from build123d import *

# Parameters (mm, degrees)
SKETCH1_R                            = 3.175
SKETCH1_R_2                          = 1.5875
BOSS_EXTRUDE1_DEPTH                  = 19.05
TAPPED_HOLE_FOR_4_40_HELICOIL2_D     = 3.048
TAPPED_HOLE_FOR_4_40_HELICOIL2_DEPTH = 9.6012
TAPPED_HOLE_FOR_4_40_HELICOIL2_TIP   = 0.915711583
SKETCH7_W                            = 1.190625
SKETCH7_H                            = 3.175
TAPPED_HOLE_FOR_4_40_HELICOIL3_D     = 3.048
TAPPED_HOLE_FOR_4_40_HELICOIL3_DEPTH = 9.6012
TAPPED_HOLE_FOR_4_40_HELICOIL3_TIP   = 0.915711583


with BuildPart() as part:
    # Sketch1 → Boss-Extrude1 (new body)
    with BuildSketch(Plane(origin=(0, 0, 0), x_dir=(1, 0, 0), z_dir=(0, 1, 0))):
        with Locations(Location((0, 0, 0), (0, 0, 270))):  # turned: the seam where the file's is
            Circle(SKETCH1_R)
        Circle(SKETCH1_R_2, mode=Mode.SUBTRACT)
        Circle(SKETCH1_R_2)
    extrude(amount=BOSS_EXTRUDE1_DEPTH)

    # Tapped Hole for #4-40 Helicoil2
    with Locations(Plane(origin=(0, 19.05, 0), x_dir=(1, 0, 0), z_dir=(0, 1, 0))):
        with Locations((0, 0)):
            Hole(TAPPED_HOLE_FOR_4_40_HELICOIL2_D / 2, depth=TAPPED_HOLE_FOR_4_40_HELICOIL2_DEPTH)
            with Locations((0, 0, -(TAPPED_HOLE_FOR_4_40_HELICOIL2_DEPTH + TAPPED_HOLE_FOR_4_40_HELICOIL2_TIP / 2))):  # 118° drill point
                Cone(0, TAPPED_HOLE_FOR_4_40_HELICOIL2_D / 2, TAPPED_HOLE_FOR_4_40_HELICOIL2_TIP, mode=Mode.SUBTRACT)

    # Sketch7 → 3/32 (0.09375) Diameter Hole1 (revolve, cut)
    with BuildSketch(Plane.ZX.offset(9.525)):
        with Locations((0.5953125, 1.5875)):
            Rectangle(SKETCH7_W, SKETCH7_H)
    revolve(axis=Axis((-6.35, 9.525, 0), (1, 0, 0)), mode=Mode.SUBTRACT)

    # Tapped Hole for #4-40 Helicoil3
    with Locations(Plane(origin=(0, 0, 0), x_dir=(-1, 0, 0), z_dir=(0, -1, 0))):
        with Locations((0, 0)):
            Hole(TAPPED_HOLE_FOR_4_40_HELICOIL3_D / 2, depth=TAPPED_HOLE_FOR_4_40_HELICOIL3_DEPTH)
            with Locations((0, 0, -(TAPPED_HOLE_FOR_4_40_HELICOIL3_DEPTH + TAPPED_HOLE_FOR_4_40_HELICOIL3_TIP / 2))):  # 118° drill point
                Cone(0, TAPPED_HOLE_FOR_4_40_HELICOIL3_D / 2, TAPPED_HOLE_FOR_4_40_HELICOIL3_TIP, mode=Mode.SUBTRACT)


solid = part.part
CAD build for the part. Positions are in the model's coordinates, mm. Give positions to 0.01 mm unless a question says otherwise; leave off trailing zeros. Order: outer loops, then holes, each group sorted by start corner. A loop starts at its lowest first (then second) coordinate and runs counter-clockwise, first axis right, second up. Notation, with made-up numbers: (3, 87.25) -> (51, 87.25) arc R31 cw to (51, 120.25) -> close; hole circle Ø1 at (28.25, 36). An arc over 180 degrees is marked (long way). Return JSON: item names as keys, results as strings.
Q1. Saw through at A-A (x = 0). Write the cut outline in (y, z) (3 decimals), then the cut area to 3 significant figures.
Working result:
{"outline": "(0, -3.175) -> (19.05, -3.175) -> (19.05, -1.524) -> (0, -1.524) -> close; (0, 1.524) -> (19.05, 1.524) -> (19.05, 3.175) -> (0, 3.175) -> close", "area": "62.9 mm²"}
Q2. Saw through at B-B (z = 0). Write the cut outline in (x, y) (3 decimals), then the cut area to 3 significant figures.
Working result:
{"outline": "(-3.175, 0) -> (-1.524, 0) -> (-1.524, 19.05) -> (-3.175, 19.05) -> close; (1.524, 0) -> (3.175, 0) -> (3.175, 8.334) -> (1.524, 8.334) -> close; (1.524, 10.716) -> (3.175, 10.716) -> (3.175, 19.05) -> (1.524, 19.05) -> close", "area": "59.0 mm²"}
Q3. Saw through at C-C (x = 2). Write the cut outline in (y, z) (3 decimals), then the cut area to 3 significant figures.
Working result:
{"outline": "(0, -2.466) -> (19.05, -2.466) -> (19.05, 2.466) -> (0, 2.466) -> close; hole circle Ø2.381 at (9.525, 0)", "area": "89.5 mm²"}
Q4. Flat gauge pin, fed straight in: pin 1 (1 mm diameter, centred on x = 2.5, y = 7.5, fed in from -Z). Where does the tip first touch, or does it go through?
Working result:
{"pin 1": "z = -2.47"}
Q5. Saw through at D-D (y = 6.5). Write the cut outline in (x, z) (3 decimals), then the cut area to 3 significant figures.
Working result:
{"outline": "circle Ø6.35 at (0, 0); hole circle Ø3.048 at (0, 0)", "area": "24.4 mm²"}
Q6. Mould opens along Y. For faces 1 (the face through (2.08, 9.98, 1.1)), 2 (the face through (-1.37, 9.66, 0.67)), 3 (the face through (1.5, 0, -0.8)), 4 (the face through (1.5, 19.05, -0.8)) say: pulls with the +Y half, pulls with the -Y half, needs draft (parallel to the pull), parting line crosses it, or undercut.
Working result:
{"face 1": "undercut", "face 2": "needs draft", "face 3": "pulls with the -Y half", "face 4": "pulls with the +Y half"}
Q7. Drill centre lines: line 1 (Y direction, x = 2.7, z = 0); line 2 (Z direction, x = 0.5, y = 10.25); line 3 (Z direction, x = 1, y = 4.5). Where is each one in solid material? Low to high.
Working result:
{"line 1": "0 to 8.33, 10.72 to 19.05", "line 2": "-3.14 to -1.44, 1.44 to 3.14", "line 3": "-3.01 to -1.15, 1.15 to 3.01"}
